Model file for the job. Use its own axes, mm. A direction names the side the tool comes from. Round coordinates to 2 decimals unless told otherwise and drop trailing zeros. Order: outer loops, then holes, each group sorted by start corner. A loop starts at its lowest first (then second) coordinate and runs counter-clockwise, first axis right, second up. Notation, with made-up numbers: M 5,19.5 L 62,19.5 A18 cw 62,37.5 Z; hole C 77.5,44 d8. An arc over 180 degrees is marked long. Return JSON: item names as keys, results as strings. Group by question number.
Item 1: Slice it at C-C on x = 20.5. Write the cut outline in (y, z) (3 decimals), then the cut area to 3 significant figures.
Item 2: Slice it at B-B on z = -2. Write the cut outline in (x, y), then the cut area to 3 significant figures.
Item 3: Which spindle directions (+Z, -Z, +X, -X, +Y, -Y) get a long thin tool onto all of the face, cutting with end or side? Do faces 5 (the face through (19, 32, -21.095)), 6 (the face through (19, 19.8, -23)), 7 (the face through (11.6, 12.8, -22.9)). Say none if no direction does.
Item 4: Slice it at A-A on y = 3. Give the number of separate pieces and of enclosed holes in the cut face, then the cut area to 3 significant figures.
Item 5: Pull direction X, two halves, no side cores. Call faces 1 (the face through (4.6, 32.3, -22.8)), 2 (the face through (37.2, 14, -20)), 3 (the face through (19, 23, -18.345)), 4 (the face through (4.6, 27, -23)): pulls with the +X half, pulls with the -X half, needs draft (parallel to the pull), parting line crosses it, or undercut.
Item 6: Probe line 1 along Z through (x, y) = (6.8, 4) (1 decimal); line 2 along Z through (x, y) = (7.5, 34) (3 decimals); line 3 along X through (y, z) = (9.5, -6.5). List the from-to ranges inside material, lowest first.
Item 7: Slice it at D-D on y = 33.5. Write the cut outline in (x, z) (3 decimals), then the cut area to 3 significant figures.
Item 8: Pin check, flat tips, straight feed: pin 1 Ø7 at (x, z) = (34, -10) entering from +Y; pin 2 Ø5 at (x, z) = (17.5, -3.5) entering from +Y; pin 3 Ø12 at (x, y) = (32.5, 25.5) entering from +Z (3 decimals); pin 4 Ø2.5 at (x, z) = (19.5, -24.5) entering from -Y. Stop position of each tip, or through.
from build123d import *

# Parameters (mm, degrees)
SKETCH1_W             = 13.6
SKETCH1_H             = 27.345
BOSS_EXTRUDE1_DEPTH   = 10
BOSS_EXTRUDE1_2_DEPTH = 10
BOSS_EXTRUDE2_DEPTH   = 9
SKETCH3_R             = 1.75
CUT_EXTRUDE1_DEPTH    = 53.888836487
SKETCH6_W             = 28
SKETCH6_H             = 4
CUT_EXTRUDE2_DEPTH    = 59.422846772
CUT_EXTRUDE3_REACH    = 60.423
CUT_EXTRUDE4_START    = -9
SKETCH8_W             = 18
SKETCH8_H             = 5
CUT_EXTRUDE4_DEPTH    = 9
CHAMFER2_SIZE         = 4


with BuildPart() as part:
    # Sketch1 → Boss-Extrude1 (new body)
    with BuildSketch(Plane(origin=(0, 0, 0), x_dir=(1, 0, 0), z_dir=(0, 1, 0))):
        with Locations((6.8, 13.6725)):
            Rectangle(SKETCH1_W, SKETCH1_H)
    extrude(amount=BOSS_EXTRUDE1_DEPTH)



with BuildPart() as body_2:
    # Sketch1 → Boss-Extrude1 2 (new body)
    with BuildSketch(Plane(origin=(0, 0, 0), x_dir=(1, 0, 0), z_dir=(0, 1, 0))):
        with Locations((30.4, 13.6725)):
            Rectangle(SKETCH1_W, SKETCH1_H)
    extrude(amount=BOSS_EXTRUDE1_2_DEPTH)


with BuildPart() as part_1:
    add(part.part)

    add(body_2.part)  # Boss-Extrude2 merges body 2
    # Sketch2 → Boss-Extrude2 (add)
    with BuildSketch(Plane(origin=(0, 0, -27.345), x_dir=(-1, 0, 0), z_dir=(0, 0, -1))):
        Polygon((-37.2, 35.8), (-37.2, 10), (-31.1, 22), (-31.1, 35.8), align=None)
        Polygon((-31.1, 22), (-37.2, 10), (-31.1, 10), align=None)
        Polygon((-31.1, 35.8), (-31.1, 22), (-31.1, 10), (-23.6, 10), (-23.6, 19.8), (-13.6, 19.8), (-13.6, 10), (-6.1, 10), (-6.1, 22), (-6.1, 35.8), align=None)
        Polygon((0, 35.8), (-6.1, 35.8), (-6.1, 22), (0, 10), align=None)
        Polygon((0, 10), (-6.1, 22), (-6.1, 10), align=None)
    extrude(amount=-BOSS_EXTRUDE2_DEPTH)

    # Sketch3 → Cut-Extrude1 (cut, through all)
    with BuildSketch(Plane(origin=(0, 10, 0), x_dir=(1, 0, 0), z_dir=(0, 1, 0))):
        with Locations(Location((30.4, 9.1725, 0), (0, 0, 270))):
            Circle(SKETCH3_R)
        with Locations(Location((6.8, 9.1725, 0), (0, 0, 90))):
            Circle(SKETCH3_R)
    extrude(amount=-CUT_EXTRUDE1_DEPTH, mode=Mode.SUBTRACT)

    # Sketch6 → Cut-Extrude2 (cut, through all)
    with BuildSketch(Plane(origin=(0, 0, -27.345), x_dir=(-1, 0, 0), z_dir=(0, 0, -1))):
        with Locations((-18.6, 26.8)):
            Rectangle(SKETCH6_W, SKETCH6_H)
    extrude(amount=-CUT_EXTRUDE2_DEPTH, mode=Mode.SUBTRACT)

    # Sketch5 → Cut-Extrude3 (cut, up to next)
    with BuildSketch(Plane(origin=(0, 35.8, 0), x_dir=(1, 0, 0), z_dir=(0, 1, 0)), mode=Mode.PRIVATE) as cut_extrude3_sk1:
        with BuildLine():
            Line((6.35, 24.595), (30.85, 24.595))
            ThreePointArc((30.85, 24.595), (32.6, 22.845), (30.85, 21.095))
            Line((30.85, 21.095), (6.35, 21.095))
            ThreePointArc((6.35, 21.095), (4.6, 22.845), (6.35, 24.595))
        make_face()
    cut_extrude3_tool1 = extrude(cut_extrude3_sk1.sketch, amount=-CUT_EXTRUDE3_REACH, mode=Mode.PRIVATE) & part_1.part
    add(cut_extrude3_tool1.solids().sort_by_distance((18.6, 35.8, -22.845))[0], mode=Mode.SUBTRACT)

    # Sketch8 → Cut-Extrude4 (cut)
    with BuildSketch(Plane.XY.offset(-18.345).offset(CUT_EXTRUDE4_START)):
        with Locations((18.6, 17.3)):
            Rectangle(SKETCH8_W, SKETCH8_H)
    extrude(amount=CUT_EXTRUDE4_DEPTH, mode=Mode.SUBTRACT)

    # Chamfer2
    chamfer2_edges = [part_1.edges().sort_by_distance(p)[0] for p in [
        (27.6, 19.8, -22.845),
        (9.6, 19.8, -22.845),
    ]]
    chamfer(chamfer2_edges, length=CHAMFER2_SIZE)
    chamfer2_2_edges = [part_1.edges().sort_by_distance(p)[0] for p in [
        (23.6, 14.8, -22.845),
        (13.6, 14.8, -22.845),
    ]]
    chamfer(chamfer2_2_edges, length=CHAMFER2_SIZE - 0.0001)  # a hair under: the kernel refuses the full size


solid = part_1.part
Output values:
{
 "1": {"outline": "M 19.8,-27.345 L 24.8,-27.345 L 24.8,-18.345 L 19.8,-18.345 Z; M 28.8,-27.345 L 35.8,-27.345 L 35.8,-24.595 L 28.8,-24.595 Z; M 28.8,-21.095 L 35.8,-21.095 L 35.8,-18.345 L 28.8,-18.345 Z", "area": "83.5 mm²"},
 "2": {"outline": "M 0,0 L 13.6,0 L 13.6,10 L 0,10 Z; M 23.6,0 L 37.2,0 L 37.2,10 L 23.6,10 Z", "area": "272 mm²"},
 "3": {"face 5": "+Y", "face 6": "+Z, -Z, -Y", "face 7": "+Z, -Z"},
 "4": {"separate pieces": "2", "enclosed holes": "2", "area": "725 mm²"},
 "5": {"face 1": "undercut", "face 2": "pulls with the +X half", "face 3": "needs draft", "face 4": "undercut"},
 "6": {"line 1": "-27.3 to -10.9, -7.4 to 0", "line 2": "-27.345 to -24.595, -21.095 to -18.345", "line 3": "0 to 13.6, 23.6 to 37.2"},
 "7": {"outline": "M 0,-27.345 L 37.2,-27.345 L 37.2,-18.345 L 0,-18.345 Z; hole M 6.35,-24.595 L 30.85,-24.595 A1.75 ccw 30.85,-21.095 L 6.35,-21.095 A1.75 ccw Z", "area": "239 mm²"},
 "8": {"pin 1": "y = 10", "pin 2": "through", "pin 3": "z = -18.345", "pin 4": "y = 19.8"}
}
